The listing builds one solid part. Answer for the finished solid, in the listing's coordinates (mm). Face numbers are marked on the shaded views. Round coordinates to 2 decimals unless told otherwise and drop trailing zeros. Order: outer loops, then holes, each group sorted by start corner. A loop starts at its lowest first (then second) coordinate and runs counter-clockwise, first axis right, second up. Notation, with made-up numbers: (34, 79) - (75, 79) arc R11 ccw to (75, 99) - close; hole circle Ø6 at (60, -26.75). An arc over 180 degrees is marked (long way). Write item = value, one per line.
Autodesk Inventor part; units mm, degrees
ref_plane "YZ Plane" through (0, 0, 0) normal (1, 0, 0) x (0, 1, 0)
ref_plane "XZ Plane" through (0, 0, 0) normal (0, 1, 0) x (-1, 0, 0)
ref_plane "XY Plane" through (0, 0, 0) normal (0, 0, 1) x (1, 0, 0)
sketch "Эскиз1" plane through (0, 0, 0) normal (0, 0, 1) x (1, 0, 0)
  line L0 (0, 0) -> (6.2046, 0)
  line L1 (0, 0) -> (0, 45)
  line L2 (0, 45) -> (2.55, 45)
  line L3 (2.55, 45) -> (3.05, 44.5)
  line L4 (3.05, 44.5) -> (5.55, 44.5)
  line L5 (5.55, 44.5) -> (5.55, 48)
  line L6 (5.55, 48) -> (10.55, 48)
  line L7 (10.55, 48) -> (10.55, 35.3814)
  line L8 (10.55, 35.3814) -> (5, 35.3814)
  line L9 (5, 35.3814) -> (5, 0)
  line L10 (0, 0) -> (5, 0)
  dimension "d0" = 45
  dimension "d1" = 0.5
  dimension "d2" = 90
  dimension "d3" = 10.55
  dimension "d4" = 5
  dimension "d6" = 3
  dimension "d7" = 2.5
  dimension "d8" = 5
revolve "Вращение1" add sketch "Эскиз1" angle 360 about axis through (0, 0, 0) along (1, 0, 0)
sketch "Эскиз2" plane through (0, 0, 0) normal (-1, 0, 0) x (0, 0, 1)
  circle A0 centre (0, 0) radius 5
  dimension "d10" = 10
extrude "Выдавливание1" cut sketch "Эскиз2" against normal through all
thread "Резьба1"
chamfer "Фаска1" distance 1 angle 45 1 edges at (0, 0, -5)
sketch "Эскиз3" plane through (5, 0, 0) normal (1, 0, 0) x (0, 0, -1)
  circle A0 centre (0, 0) radius 5
  circle A1 centre (0, 0) radius 35.3814
extrude "Выдавливание2" add sketch "Эскиз3" along normal blind 3
properties part number "Крышка тих"
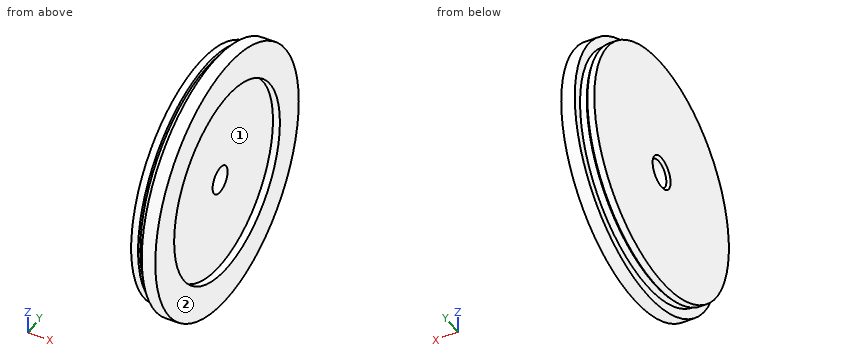
Q1. Find the intervals of material crossed by line 1 (Z direction, x = 5.75, y = 0); line 2 (Z direction, x = 5.5, y = 0); line 3 (X direction, y = 6, z = -1), in increasing order. Write a range as from..to.
Model answer:
line_1 = -48..-5, 5..48
line_2 = -44.5..-5, 5..44.5
line_3 = 0..8
Q2. Section A-A on y = 0 is taken. Determine the outline of the cut face in (x, z), then the cut area to 3 significant figures.
Model answer:
outline = (0, -45) - (2.55, -45) - (3.05, -44.5) - (5.55, -44.5) - (5.55, -48) - (10.55, -48) - (10.55, -35.38) - (8, -35.38) - (8, -5) - (1, -5) - (0, -6) - close; (0, 6) - (1, 5) - (8, 5) - (8, 35.38) - (10.55, 35.38) - (10.55, 48) - (5.55, 48) - (5.55, 44.5) - (3.05, 44.5) - (2.55, 45) - (0, 45) - close
area = 715 mm^2
Q3. Flat-ended cylindrical pins translate along their axes: P1, Ø4, axis at x = 4, z = 3.5, coming from the +Y side; P2, Ø4, axis at x = 7, z = 19, coming from the -Y side; P3, Ø2, axis at x = 7.5, y = 34, coming from the -Z side. Find the tip coordinate at first contact, or state that the pin passes through.
Model answer:
P1 = 47.95
P2 = -44.89
P3 = -34.86
Q4. Determine the mould class of the marked faces 1 and 2 for opening direction Z: released by +Z, released by -Z, zero draft, split by the parting line, or undercut.
Model answer:
face_1 = undercut
face_2 = zero draft
